Model file for the job. Use its own axes, mm. A direction names the side the tool comes from. Round coordinates to 2 decimals unless told otherwise and drop trailing zeros. Loops run counter-clockwise (first coordinate to the right, second up) from the corner with the lowest first, then second, coordinate; pieces in that order, holes last. Notation, with made-up numbers: M 86,-5 L 135,-5 A16 ccw 135,19 Z; hole C -32.75,-4.75 d11. An arc over 180 degrees is marked long. Use a Markdown table: item, result. Add a question column.
Item 1: Wall check: L1, parallel to Y at x = -7.55, z = -2.95; L2, parallel to X at y = -17.5, z = -2.8; L3, parallel to Y at x = -7, z = -8.5. Give the ranges that are in metal, low to high. Write a range as from..to.
Item 2: Pin check, flat tips, straight feed: P1, Ø5, axis at x = -8.5, z = -12.5, coming from the -Y side; P2, Ø1, axis at x = -10.5, y = 0, coming from the +Z side; P3, Ø8, axis at x = 0.5, z = -5, coming from the -Y side; P4, Ø3, axis at x = -7.55, y = 17.5, coming from the -Z side. Stop position of each tip, or through.
Item 3: Saw through at B-B on y = 0. Write the cut outline in (x, z), then the cut area to 3 significant figures.
Item 4: Saw through at D-D on x = -20. Write the cut outline in (y, z), then the cut area to 3 significant figures.
Item 5: Tool access for faces 5 (the flat face through (-22, 7.5, -14)), 6 (the flat face through (-22, -7.5, -14)), 7 (the cylindrical face through (2.385, -0.751, 3.12)), 8 (the flat face through (0, 2, 2.17)): list every direction of +Z, -Z, +X, -X, +Y, -Y with a clear straight run to the whole face (end or side of a thin tool).
Item 6: Saw through at A-A on x = -7.55. Write the cut outline in (y, z), then the cut area to 3 significant figures.
Item 7: Saw through at C-C on z = -12. Write the cut outline in (x, y), then the cut area to 3 significant figures.
Item 8: Two-plate mould, pull along X, no slides. Class faces 1 (the cylindrical face through (0.99, 4.44, -1.49)), 2 (the flat face through (-24.55, 0, -14)), 3 (the flat face through (-22, 0, -5)), 4 (the cylindrical face through (-7.81, -15.517, -2.924)): +X half, -X half, draft (parallel to the pull), parting line (faces both ways), or undercut.
Autodesk Inventor part; units mm, degrees
ref_plane "align plane" through (-7.55, 0, -2.5) normal (1, 0, 0) x (0, 1, 0)
ref_plane "XZ Plane" through (0, 0, 0) normal (0, 1, 0) x (-1, 0, 0)
ref_plane "XY Plane" through (0, 0, 0) normal (0, 0, 1) x (1, 0, 0)
sketch "Sketch1" plane through (0, 0, 0) normal (0, 0, 1) x (1, 0, 0)
  circle A0 centre (0, 0) radius 2.5
  dimension "d0" = 5
extrude "Extrusion1" add sketch "Sketch1" along normal blind 8.17
sketch "Sketch2" plane through (0, 0, 8.17) normal (0, 0, 1) x (1, 0, 0)
  circle A0 centre (0, 0) radius 2.5 construction
  circle A1 centre (0, 0) radius 2.5 construction
  line L0 (-2, -1.5) -> (2, -1.5)
  line L1 (2, -1.5) -> (2, 1.5)
  line L2 (2, 1.5) -> (-2, 1.5)
  line L3 (-2, 1.5) -> (-2, -1.5)
  line L4 (-2, -1.5) -> (2, 1.5) construction
  line L5 (2, -1.5) -> (-2, 1.5) construction
  arc A2 (-2, 1.5) -> (-2, -1.5) centre (0, 0) ccw
  arc A3 (2, 1.5) -> (-2, 1.5) centre (0, 0) ccw
  arc A4 (-2, -1.5) -> (2, -1.5) centre (0, 0) ccw
  arc A5 (2, -1.5) -> (2, 1.5) centre (0, 0) ccw
  dimension "d3" = 3
extrude "Extrusion2" cut sketch "Sketch2" against normal blind 6 contours L0 A4 | A3 L2
sketch "Sketch3" plane through (0, 0, 0) normal (0, 0, -1) x (-1, 0, 0)
  circle A0 centre (0, 0) radius 2.5
  circle A1 centre (0, 0) radius 4.55
  dimension "d6" = 9.1
extrude "Extrusion3" add sketch "Sketch3" along normal blind 2.5 contours A0 | A1
sketch "Sketch4" plane through (0, 0, -2.5) normal (0, 0, -1) x (-1, 0, 0)
  circle A0 centre (7.55, 0) radius 14
  circle A1 centre (0, 0) radius 4.55
  line L0 (4.55, 0) -> (-6.45, 0) construction
  dimension "d9" = 28
  dimension "d10" = 11
extrude "Extrusion4" add sketch "Sketch4" along normal blind 19.3 contours A0 | A1
fillet "Fillet1" radius 0.5 1 edges at (4.55, 0, 0)
sketch "Sketch5" plane through (-7.55, 0, -21.8) normal (0, 0, -1) x (-1, 0, 0)
  circle A0 centre (0, 0) radius 14 construction
  line L0 (11.8216, -7.5) -> (17, -7.5)
  line L1 (17, -7.5) -> (17, 7.5)
  line L2 (17, 7.5) -> (11.8216, 7.5)
  line L3 (11.8216, 7.5) -> (11.8216, -7.5)
  line L4 (11.8216, -7.5) -> (17, 7.5) construction
  line L5 (17, -7.5) -> (11.8216, 7.5) construction
  circle A1 centre (0, 0) radius 14 construction
  line L6 (17, 0) -> (-14, 0) construction
  circle A2 centre (0, 0) radius 14 construction
  point P0 (-7.55, 0)
  point P1 (14.4108, 0)
  dimension "d14" = 15
  dimension "d15" = 31
extrude "Extrusion5" add sketch "Sketch5" against normal blind 16.8
sketch "Sketch6" plane through (-7.55, 0, -2.5) normal (0, 0, 1) x (1, 0, 0)
  circle A0 centre (0, 0) radius 14
  circle A1 centre (7.55, 0) radius 4.55 construction
  arc A2 (-11.8216, -7.5) -> (-11.8216, 7.5) centre (0, 0) ccw
  line L0 (3.55, 13.5424) -> (3.55, 17.5)
  arc A3 (3.55, 17.5) -> (-3.55, 17.5) centre (0, 17.5) ccw
  line L1 (-3.55, 17.5) -> (-3.55, 13.5424)
  circle A4 centre (0, 17.5) radius 2
  dimension "d18" = 4
  dimension "d19" = 7.1
  dimension "d20" = 17.5
extrude "Extrusion6" add sketch "Sketch6" against normal blind 0.86 contours A0 L1 A3 L0
mirror "Mirror1" about plane through (0, 0, 0) normal (0, 1, 0) of "Extrusion6"
sketch "Sketch7" plane through (0, 0, -2.5) normal (0, 0, 1) x (1, 0, 0)
  arc A0 (-4, -13.5424) -> (-4, 13.5424) centre (-7.55, 0) ccw
  point P0 (0, 0)
ref_plane "align plane" through (-7.55, 0, -2.5) normal (1, 0, 0) x (0, 1, 0)
properties part number "stepper motor-cheapo geared"
Entries:
| question | item | result |
|---|---|---|
| 1 | L1 | -21.05..-19.5, -15.5..15.5, 19.5..21.05 |
| 1 | L2 | -11.1..-9.55, -5.55..-4 |
| 1 | L3 | -13.99..13.99 |
| 2 | P1 | y = -14 |
| 2 | P2 | z = -2.5 |
| 2 | P3 | y = -13.4 |
| 2 | P4 | through |
| 3 | outline | M -24.55,-21.8 L 6.45,-21.8 L 6.45,-2.5 L 4.55,-2.5 L 4.55,-0.5 A0.5 ccw 4.05,0 L 2.5,0 L 2.5,8.17 L -2.5,8.17 L -2.5,0 L -4.05,0 A0.5 ccw -4.55,-0.5 L -4.55,-2.5 L -21.55,-2.5 L -21.55,-5 L -24.55,-5 Z |
| 3 | area | 654 mm2 |
| 4 | outline | M -7.5,-21.8 L 7.5,-21.8 L 7.5,-5 L 6.4,-5 L 6.4,-2.5 L -6.4,-2.5 L -6.4,-5 L -7.5,-5 Z |
| 4 | area | 284 mm2 |
| 5 | face 5 | +Z, -Z, -X, +Y |
| 5 | face 6 | +Z, -Z, -X, -Y |
| 5 | face 7 | +Z |
| 5 | face 8 | +Z, +X, -X, +Y |
| 6 | outline | M -21.05,-3.36 L -19.5,-3.36 L -19.5,-2.5 L -21.05,-2.5 Z; M -15.5,-3.36 L -14,-3.36 L -14,-21.8 L 14,-21.8 L 14,-3.36 L 15.5,-3.36 L 15.5,-2.5 L -15.5,-2.5 Z; M 19.5,-3.36 L 21.05,-3.36 L 21.05,-2.5 L 19.5,-2.5 Z |
| 6 | area | 546 mm2 |
| 7 | outline | M -24.55,-7.5 L -19.37,-7.5 A14 ccw long -19.37,7.5 L -24.55,7.5 Z |
| 7 | area | 671 mm2 |
| 8 | face 1 | parting line |
| 8 | face 2 | -X half |
| 8 | face 3 | draft |
| 8 | face 4 | undercut |
